```python
from build123d import *

# Parameters (mm, degrees)
SKETCH1_W                             = 28
SKETCH1_H                             = 46
SKETCH1_R                             = 2
BOSS_EXTRUDE1_DEPTH                   = 8
SKETCH6_R                             = 2.25
DRAGCHAINMOUNTHOLESCUT_EXTRUDE1_DEPTH = 4
SKETCH2_W                             = 28
SKETCH2_H                             = 8
BRIDGEBOSS_EXTRUDE2_DEPTH             = 7
GROMMETCUT_EXTRUDE3_DEPTH             = 40.217343102
BRIDGEMOUNTHOLESSKETCH4_R             = 2.25
BRIDGEMOUNTHOLESCUT_EXTRUDE4_DEPTH    = 4
SKETCH5_W                             = 15
SKETCH5_H                             = 4
EDGECUT_EXTRUDE5_DEPTH                = 56.901699437
CHAMFER1_SIZE                         = 4


with BuildPart() as part:
    # Sketch1 → Boss-Extrude1 (new body)
    with BuildSketch(Plane(origin=(0, 0, 0), x_dir=(1, 0, 0), z_dir=(0, 1, 0))):
        with Locations((14, 23)):
            Rectangle(SKETCH1_W, SKETCH1_H)
        with Locations(Location((14, 38.5, 0), (0, 0, 270))):
            Circle(SKETCH1_R, mode=Mode.SUBTRACT)
    extrude(amount=BOSS_EXTRUDE1_DEPTH)

    # Sketch6 → DragChainMountHolesCut-Extrude1 (cut)
    with BuildSketch(Plane(origin=(0, 8, 0), x_dir=(1, 0, 0), z_dir=(0, 1, 0))):
        with Locations(Location((8, 16, 0), (0, 0, 270))):
            Circle(SKETCH6_R)
        with Locations(Location((19.996983409, 16, 0), (0, 0, 270))):
            Circle(SKETCH6_R)
        with Locations(Location((14, 10, 0), (0, 0, 270))):
            Circle(SKETCH6_R)
    extrude(amount=-DRAGCHAINMOUNTHOLESCUT_EXTRUDE1_DEPTH, mode=Mode.SUBTRACT)

    # Sketch2 → BridgeBoss-Extrude2 (add)
    with BuildSketch(Plane(origin=(0, 8, 0), x_dir=(1, 0, 0), z_dir=(0, 1, 0))):
        with Locations((14, 27)):
            Rectangle(SKETCH2_W, SKETCH2_H)
    extrude(amount=BRIDGEBOSS_EXTRUDE2_DEPTH)

    # Sketch3 → GrommetCut-Extrude3 (cut, through all)
    with BuildSketch(Plane.XY.offset(-23)):
        with BuildLine():
            Line((9.75, 15), (18.25, 15))
            ThreePointArc((18.25, 15), (14, 10.75), (9.75, 15))
        make_face()
    extrude(amount=-GROMMETCUT_EXTRUDE3_DEPTH, mode=Mode.SUBTRACT)

    # BridgeMountHolesSketch4 → BridgeMountholesCut-Extrude4 (cut)
    with BuildSketch(Plane(origin=(0, 15, 0), x_dir=(1, 0, 0), z_dir=(0, 1, 0))):
        with Locations(Location((4.875, 27, 0), (0, 0, 270))):
            Circle(BRIDGEMOUNTHOLESSKETCH4_R)
        with Locations(Location((23.125, 27, 0), (0, 0, 270))):
            Circle(BRIDGEMOUNTHOLESSKETCH4_R)
    extrude(amount=-BRIDGEMOUNTHOLESCUT_EXTRUDE4_DEPTH, mode=Mode.SUBTRACT)

    # Sketch5 → EdgeCut-Extrude5 (cut, through all)
    with BuildSketch(Plane.ZY):
        with Locations((-38.5, 2)):
            Rectangle(SKETCH5_W, SKETCH5_H)
    extrude(amount=-EDGECUT_EXTRUDE5_DEPTH, mode=Mode.SUBTRACT)

    # Chamfer1
    chamfer1_edges = [part.edges().sort_by_distance(p)[0] for p in [
        (28, 8, -38.5),
        (0, 8, -38.5),
    ]]
    chamfer(chamfer1_edges, length=CHAMFER1_SIZE - 0.0001)  # a hair under: the kernel refuses the full size


solid = part.part
```
Geometry check sheet. Reference: the model listing, model coordinates, mm. A direction names the side the tool comes from. Coordinates: 2 decimals unless noted, no trailing zeros. Write each loop counter-clockwise with the first axis right and the second up, starting at its lowest first coordinate (ties: lowest second). Pieces come first, ordered by that corner, then holes. Notation, with made-up numbers: M -29,10 L 8,10 A25 ccw 8,23 Z; hole C -30,48.5 d5. An arc over 180 degrees is marked long. Use one line per item in the form item = value. Start each with the question number.
1) Set-up check for faces 4 (the flat face through (11.6, 8, -38.6)), 5 (the cylindrical face through (12.631, 6.028, -11.786)), 6 (the flat face through (14, 8, -14)): record each of +Z, -Z, +X, -X, +Y, -Y from which the full face is reachable in a straight line by a thin tool's end or side.
2) Section check D-D on z = -16. Enter the section's corners in (x, y), and give its area (3 significant figures).
3) Section check C-C on x = 14. Enter the section's corners in (y, z).
4) Section check B-B on y = 12. Enter the section's corners in (x, z) (3 decimals), and give its area (3 significant figures).
5) Release check for a two-part mould opening along Z. For faces 1 (the flat face through (11, 4, -39)), 2 (the flat face through (8, 4, -16)), 3 (the flat face through (14, 4, 0)) record: pulls with the +Z half, pulls with the -Z half, needs draft (parallel to the pull), parting line crosses it, or undercut.
6) Go/stop test with flat-tipped pins: pin 1 Ø7.5 at (x, y) = (13, 12.5) entering from +Z; pin 2 Ø11.5 at (x, z) = (8, -10.5) entering from +Y; pin 3 Ø2 at (x, z) = (9, -16) entering from +Y. Record where each tip stops, or that it passes through.
7) Thickness scan on probe 1 along X at (y, z) = (13.75, -27) (3 decimals); probe 2 along X at (y, z) = (13.6, -27) (3 decimals); probe 3 along X at (y, z) = (6.7, -10). Record the ranges inside material, lowest first. Write a range as from..to.
Responses:
q1.face_4 = -Z, +X, -X, +Y
q1.face_5 = +Y
q1.face_6 = +Z, +X, -X, +Y
q2.outline = M 0,0 L 28,0 L 28,8 L 22.25,8 L 22.25,4 L 17.75,4 L 17.75,8 L 10.25,8 L 10.25,4 L 5.75,4 L 5.75,8 L 0,8 Z
q2.area = 188 mm2
q3.outline = M 0,-31 L 4,-31 L 4,-36.5 L 8,-36.5 L 8,-31 L 10.75,-31 L 10.75,-23 L 8,-23 L 8,-12.25 L 4,-12.25 L 4,-7.75 L 8,-7.75 L 8,0 L 0,0 Z; M 4,-46 L 8,-46 L 8,-40.5 L 4,-40.5 Z
q4.outline = M 0,-31 L 10.99,-31 L 10.99,-23 L 0,-23 Z; M 17.01,-31 L 28,-31 L 28,-23 L 17.01,-23 Z; hole C 4.875,-27 d4.5; hole C 23.125,-27 d4.5
q4.area = 144 mm2
q5.face_1 = needs draft
q5.face_2 = undercut
q5.face_3 = pulls with the +Z half
q6.pin_1 = -23
q6.pin_2 = 8
q6.pin_3 = 4
q7.probe_1 = 0..2.625, 7.125..9.938, 18.062..20.875, 25.375..28
q7.probe_2 = 0..2.625, 7.125..9.987, 18.013..20.875, 25.375..28
q7.probe_3 = 0..11.75, 16.25..28
